Autodesk Inventor part; units mm, degrees
ref_plane "YZ Plane" through (0, 0, 0) normal (1, 0, 0) x (0, 1, 0)
ref_plane "XZ Plane" through (0, 0, 0) normal (0, 1, 0) x (-1, 0, 0)
sketch "Sketch1" plane through (0, 0, 0) normal (0, 1, 0) x (-1, 0, 0)
  line L0 (-40, -23) -> (0, -23)
  line L1 (-40, 23) -> (0, 23)
  line L2 (0, 23) -> (0, -23)
  line L3 (-40, 23) -> (-40, -23)
  line L4 (-40, -12) -> (0, -12) construction
  line L5 (-40, 12) -> (0, 12) construction
  line L6 (-4, 23) -> (-4, -23) construction
  circle A0 centre (-9.5, 12) radius 3.5 construction
  line L7 (0, 19) -> (-40, 19) construction
  point P0 (0, 0)
  dimension "d5" = 46
  dimension "d6" = 23
  dimension "d7" = 40
  dimension "d8" = 0
  dimension "d9" = 12
  dimension "d10" = 12
  dimension "d12" = 4
  dimension "d22" = 7
  dimension "d23" = 4
extrude "Lift Attachment Plate" add sketch "Sketch1" along normal blind 4
sketch "Sketch2" plane through (0, 4, 0) normal (0, 1, 0) x (1, 0, 0)
  line L0 (0, 23) -> (0, -23)
  line L1 (40, 23) -> (0, 23)
  line L2 (0, -23) -> (4, -23)
  line L3 (4, -23) -> (4, 23)
  line L4 (4, 23) -> (0, 23)
  line L5 (0, 23) -> (0, -23)
  point P0 (0, 0)
  dimension "d26" = 4
extrude "Cross bar Attachment Plate" add sketch "Sketch2" along normal blind 44
sketch "Sketch3" plane through (0, 0, 23) normal (0, 0, 1) x (1, 0, 0)
  line L0 (4, 4) -> (4, 48)
  line L1 (4, 48) -> (4, 4)
  line L2 (40, 4) -> (4, 4)
  line L3 (4, 4) -> (40, 4)
  line L4 (40, 4) -> (4, 48)
  point P0 (0, 0)
extrude "Left bracket" add sketch "Sketch3" against normal blind 4
sketch "Sketch4" plane through (0, 0, 0) normal (0, 0, 1) x (1, 0, 0)
  line L0 (4, 48) -> (40, 4)
  line L1 (4, 4) -> (40, 4)
  line L2 (4, 48) -> (4, 4)
  line L3 (4, 4) -> (40, 4)
  line L4 (40, 4) -> (4, 48)
  point P0 (0, 0)
extrude "Center bracket" add sketch "Sketch4" along normal mid plane 10
sketch "Sketch5" plane through (40, 0, -23) normal (0, 0, -1) x (-1, 0, 0)
  line L0 (36, 48) -> (40, 48)
  line L1 (36, 48) -> (36, 4)
  line L2 (36, 48) -> (36, 4)
  line L3 (0, 4) -> (36, 4)
  line L4 (36, 4) -> (0, 4)
  line L5 (0, 4) -> (36, 48)
  point P0 (40, 0)
extrude "Right bracket" add sketch "Sketch5" against normal blind 4
sketch "Sketch6" plane through (0, 0, -23) normal (-1, 0, 0) x (0, 0, 1)
  circle A0 centre (35, 11) radius 2 construction
  circle A1 centre (11, 11) radius 2 construction
  line L0 (0, 0) -> (46, 0) construction
  line L1 (23, 57.6) -> (23, -9.6) construction
  circle A2 centre (35, 43) radius 2 construction
  circle A3 centre (11, 43) radius 2 construction
  line L2 (42, 48) -> (42, 4) construction
  line L3 (4, 4) -> (4, 48) construction
  line L4 (15, 11) -> (7, 11) construction
  line L5 (4, 4) -> (4, 48)
  line L6 (12.8, 13.2) -> (9.2, 13.2)
  line L7 (9.2, 8.8) -> (12.8, 8.8)
  arc A4 (12.8, 8.8) -> (12.8, 13.2) centre (12.8, 11) ccw
  arc A5 (9.2, 13.2) -> (9.2, 8.8) centre (9.2, 11) ccw
  point P0 (23, 0)
  dimension "d35" = 4
  dimension "d36" = 4
  dimension "d37" = 11
  dimension "d38" = 11
  dimension "d39" = 12
  dimension "d40" = 12
  dimension "d41" = 4
  dimension "d42" = 4
  dimension "d43" = 32
  dimension "d44" = 32
  dimension "d45" = 4
  dimension "d46" = 4
  dimension "d47" = 4.4
extrude "Extrusion6" cut sketch "Sketch6" against normal through all
pattern_linear "Rectangular Pattern1" count 2 spacing 24 along (0, 0, 1) count 2 spacing 32 along (0, 1, 0) of "Extrusion6"
sketch "Sketch7" plane through (0, 4, 0) normal (0, 1, 0) x (1, 0, 0)
  circle A0 centre (13.4704, -13.4704) radius 1.778 construction
  circle A1 centre (24.6296, -13.4704) radius 1.778 construction
  circle A2 centre (32.5204, -13.4704) radius 1.778 construction
  circle A3 centre (24.6296, 13.4704) radius 1.778 construction
  circle A4 centre (13.4704, 13.4704) radius 1.778 construction
  circle A5 centre (32.5204, 13.4704) radius 1.778 construction
  circle A6 centre (13.4704, -13.4704) radius 2.032
  circle A7 centre (24.6296, -13.4704) radius 2.032
  circle A8 centre (32.5204, -13.4704) radius 2.032
  circle A9 centre (13.4704, 13.4704) radius 2.032
  circle A10 centre (24.6296, 13.4704) radius 2.032
  circle A11 centre (32.5204, 13.4704) radius 2.032
  point P0 (0, 0)
  dimension "d56" = 4.064
  dimension "d57" = 4.064
  dimension "d58" = 4.064
  dimension "d59" = 4.064
  dimension "d60" = 4.064
  dimension "d61" = 4.064
extrude "Extrusion7" cut sketch "Sketch7" against normal blind 10
equation "\"d38\" = d37"
equation "\"d39\" = d40"
equation "\"d44\" = d43"
equation "\"d46\" = d45"
properties part number "Cross bar bracket actobotics"
Check sheet for the modelled part. Datum: model origin and axes. Units: mm. A direction names the side the tool comes from. Round coordinates to 2 decimals unless told otherwise and drop trailing zeros. Order: outer loops, then holes, each group sorted by start corner. A loop starts at its lowest first (then second) coordinate and runs counter-clockwise, first axis right, second up. Notation, with made-up numbers: (40.25, -24.5) - (78.25, -24.5) arc R15 cw to (78.25, 0.5) - close; hole circle Ø10 at (75.5, 3.5). An arc over 180 degrees is marked (long way). Write item = value, one per line.
Q1. Thickness scan on line 1 along Z through (x, y) = (15.5, 33); line 2 along X through (y, z) = (20.5, 9.5). Record the ranges inside material, lowest first.
Computed:
line_1 = -23 to -19, -5 to 5, 19 to 23
line_2 = 0 to 4
Q2. Go/stop test with flat-tipped pins: pin 1 (5.5 mm diameter, centred on x = 13.47, z = 13.47, fed in from -Y); pin 2 (1.5 mm diameter, centred on y = 21.5, z = 8, fed in from +X); pin 3 (4 mm diameter, centred on x = 13.5, z = 16.5, fed in from +Y); pin 4 (15.5 mm diameter, centred on x = 22, z = 12.5, fed in from +Y). Record where each tip stops, or that it passes through.
Computed:
pin_1 = 0
pin_2 = 4
pin_3 = 4
pin_4 = 31.16
Q3. Section check C-C (z = -6.5). Record the boundary of the cut face in (x, y).
Computed:
outline = (0, 0) - (40, 0) - (40, 4) - (4, 4) - (4, 48) - (0, 48) - close
Q4. Section check B-B (y = 11). Record the boundary of the cut face in (x, z).
Computed:
outline = (0, -23) - (34.27, -23) - (34.27, -19) - (4, -19) - (4, -16) - (0, -16) - close; (0, -8) - (4, -8) - (4, -5) - (34.27, -5) - (34.27, 5) - (4, 5) - (4, 8) - (0, 8) - close; (0, 16) - (4, 16) - (4, 19) - (34.27, 19) - (34.27, 23) - (0, 23) - close
Q5. Draft check along Y on faces 4 (the face through (2, 40.8, 12)), 5 (the face through (2, 43, 8)), 6 (the face through (14, 17, 19)). Enter one of: pulls with the +Y half, pulls with the -Y half, needs draft (parallel to the pull), parting line crosses it, or undercut.
Computed:
face_4 = undercut
face_5 = undercut
face_6 = needs draft
Q6. Section check D-D (y = 32.5). Record the boundary of the cut face in (x, z), and give its area (3 significant figures).
Computed:
outline = (0, -23) - (16.68, -23) - (16.68, -19) - (4, -19) - (4, -5) - (16.68, -5) - (16.68, 5) - (4, 5) - (4, 19) - (16.68, 19) - (16.68, 23) - (0, 23) - close
area = 412 mm^2
Q7. Section check A-A (x = 33). Record the boundary of the cut face in (y, z) (3 decimals).
Computed:
outline = (0, -23) - (12.556, -23) - (12.556, -19) - (4, -19) - (4, -15.445) - (0, -15.445) - close; (0, -11.496) - (4, -11.496) - (4, -5) - (12.556, -5) - (12.556, 5) - (4, 5) - (4, 11.496) - (0, 11.496) - close; (0, 15.445) - (4, 15.445) - (4, 19) - (12.556, 19) - (12.556, 23) - (0, 23) - close
Q8. Tool access check on faces 1 (the face through (2, 11, -8)), 2 (the face through (14, 17, 5)), 3 (the face through (26.568, 2.028, 12.86)). Record the directions out of +Z, -Z, +X, -X, +Y, -Y that give a thin tool (end or side, any length) a straight path to the whole face; none if there is none.
Computed:
face_1 = +X, -X
face_2 = +X, +Y
face_3 = +Y, -Y
